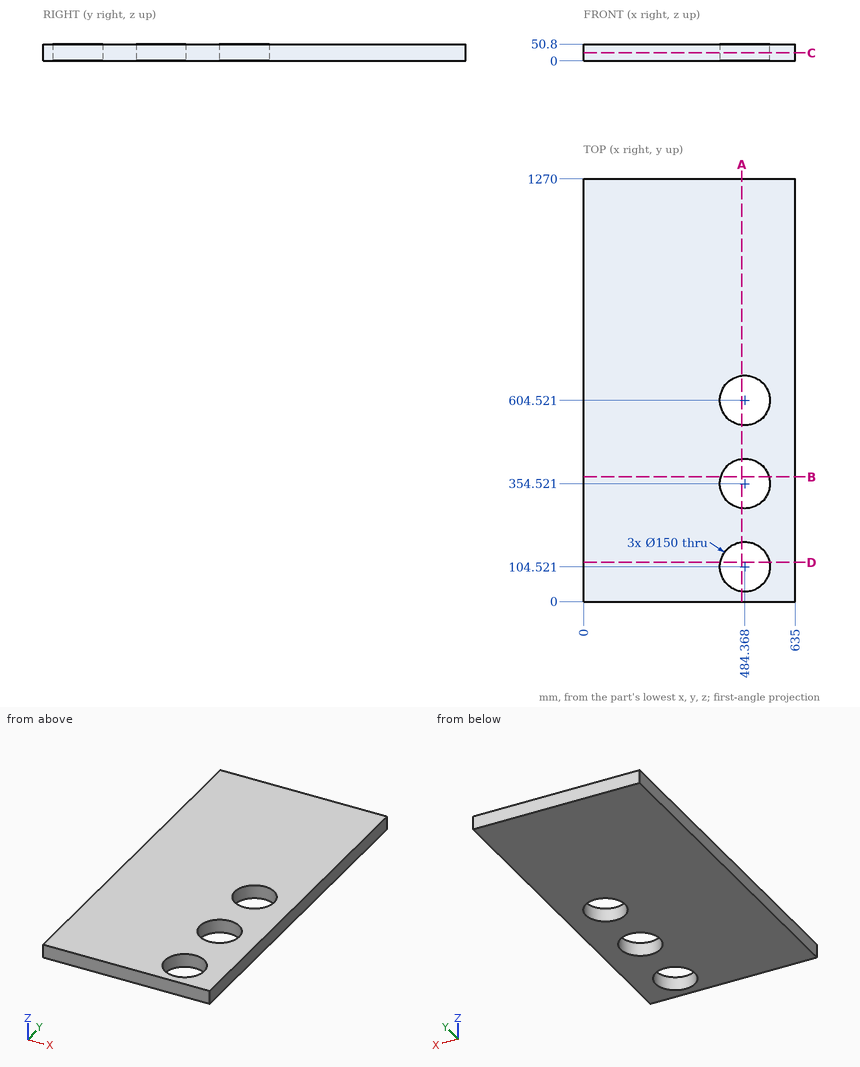
Here's the drawing with two shaded views (mm, measured from the low corner). I have some questions. Give positions to 0.01 mm unless a question says otherwise; leave off trailing zeros. Write each loop counter-clockwise with the first axis right and the second up, starting at its lowest first coordinate (ties: lowest second). Pieces come first, ordered by that corner, then holes. Notation, with made-up numbers: (-11.5, 25) - (39.5, 25) arc R7 ccw to (39.5, 37) - close; hole circle Ø7 at (-22.5, 54). An arc over 180 degrees is marked (long way). Write item = value, one per line. Start each with the question number.
1. Imagine slicing it at C-C (z = 24). Please give me the cut outline in (x, y).
2. Imagine slicing it at B-B (y = 375). Please give me the cut outline in (x, z), and give its area (3 significant figures).
3. Please list where these lines run through material, in increasing order: line 1 (X direction, y = 80, z = 26.5) (1 decimal); line 2 (X direction, y = 317.5, z = 18.5) (1 decimal).
4. Imagine slicing it at D-D (y = 117.5). Please give me the cut outline in (x, z).
5. Imagine slicing it at A-A (x = 475.5). Please give me the cut outline in (y, z) (1 decimal), and give its area (3 significant figures).
Worked answers:
q1.outline = (0, 0) - (635, 0) - (635, 1270) - (0, 1270) - close; hole circle Ø150 at (484.37, 104.52); hole circle Ø150 at (484.37, 354.52); hole circle Ø150 at (484.37, 604.52)
q2.outline = (0, 0) - (412.22, 0) - (412.22, 50.8) - (0, 50.8) - close; (556.52, 0) - (635, 0) - (635, 50.8) - (556.52, 50.8) - close
q2.area = 24,900 mm2
q3.line_1 = 0 to 413.5, 555.2 to 635
q3.line_2 = 0 to 419.1, 549.6 to 635
q4.outline = (0, 0) - (410.5, 0) - (410.5, 50.8) - (0, 50.8) - close; (558.24, 0) - (635, 0) - (635, 50.8) - (558.24, 50.8) - close
q5.outline = (0, 0) - (30, 0) - (30, 50.8) - (0, 50.8) - close; (179, 0) - (280, 0) - (280, 50.8) - (179, 50.8) - close; (429, 0) - (530, 0) - (530, 50.8) - (429, 50.8) - close; (679, 0) - (1270, 0) - (1270, 50.8) - (679, 50.8) - close
q5.area = 41,800 mm2
